The model under review builds one solid part; all positions refer to its coordinate system, in mm. A direction names the side the tool comes from. Give positions to 0.01 mm unless a question says otherwise; leave off trailing zeros. Loops run counter-clockwise (first coordinate to the right, second up) from the corner with the lowest first, then second, coordinate; pieces in that order, holes last. Notation, with made-up numbers: M -5.5,2 L 7.5,2 A4 ccw 7.5,8 Z; hole C 7.25,37.5 d2. An arc over 180 degrees is marked long. Write item = value, one per line. Start each with the question number.
1. Draft analysis for pull direction Z (two halves, no side actions). For faces 4 (the face through (48.1, 4.24, -15.86)), 5 (the face through (29, 5, -5)), 6 (the face through (6, 5, -20)), 7 (the face through (28.521, 1.774, -18.845)), state which applies: pulls with the +Z half, pulls with the -Z half, needs draft (parallel to the pull), parting line crosses it, or undercut.
2. We need section A-A on x = 53.5. Give the boundary of the cut face in (y, z), then the cut area to 4 significant figures.
3. Wall thickness on line 1 along X through (y, z) = (1.95, -20); line 2 along Y through (x, z) = (5, -16.75); line 3 along Z through (x, y) = (4, 1): over which ranges is each line inside the solid? List them lowest first. Write a range as from..to.
4. We need section D-D on x = 44. Give the boundary of the cut face in (y, z).
5. We need section B-B on z = -20. Give the boundary of the cut face in (x, y), then the cut area to 3 significant figures.
6. We need section C-C on y = 2. Give the boundary of the cut face in (x, z), then the cut area to 3 significant figures.
7. For faces 1 (the face through (45.054, 1.774, -19.328)), 2 (the face through (29, 7, -15)), 3 (the face through (52, 5, -20)), list the 3-axis set-ups (+Z, -Z, +X, -X, +Y, -Y) from which the entire face can be reached by the end or side of a thin tool; tool diameter is ignored.
8. For pin 1 (3 mm diameter, centred on x = 32.5, y = 6.5, fed in from -Z); pin 2 (11 mm diameter, centred on x = 7, z = -22, fed in from +Y); pin 3 (1.5 mm diameter, centred on x = 53.5, z = -20, fed in from +Y); pin 4 (1.5 mm diameter, centred on x = 26, y = 6, fed in from +Z), all flat-tipped, find the tip position at first contact; note any pin that passes through.
from build123d import *

# Parameters (mm, degrees)
BOSS_EXTRUDE1_DEPTH = 58
SKETCH3_W           = 40
SKETCH3_H           = 10
CUT_EXTRUDE2_DEPTH  = 6.5
CUT_EXTRUDE3_REACH  = 65.492
SKETCH4_R           = 1.25
SKETCH5_W           = 58
SKETCH5_H           = 10
CUT_EXTRUDE4_DEPTH  = 5
CUT_EXTRUDE5_REACH  = 65.356
SKETCH6_R           = 1.25
FILLET1_R           = 3


with BuildPart() as part:
    # Sketch1 → Boss-Extrude1 (new body)
    with BuildSketch(Plane(origin=(0, 0, 0), x_dir=(0, 0, -1), z_dir=(1, 0, 0))):
        Polygon((0, 0), (10, 10), (25, 10), (25, 0), align=None)
    extrude(amount=BOSS_EXTRUDE1_DEPTH)

    # Sketch3 → Cut-Extrude2 (cut)
    with BuildSketch(Plane(origin=(0, 10, 0), x_dir=(1, 0, 0), z_dir=(0, 1, 0))):
        with Locations((29, 20)):
            Rectangle(SKETCH3_W, SKETCH3_H)
    extrude(amount=-CUT_EXTRUDE2_DEPTH, mode=Mode.SUBTRACT)

    # Sketch4 → Cut-Extrude3 (cut, up to next)
    with BuildSketch(Plane(origin=(0, 3.5, 0), x_dir=(1, 0, 0), z_dir=(0, 1, 0)), mode=Mode.PRIVATE) as cut_extrude3_sk1:
        with Locations(Location((14, 20, 0), (0, 0, 270))):
            Circle(SKETCH4_R)
    cut_extrude3_tool1 = extrude(cut_extrude3_sk1.sketch, amount=-CUT_EXTRUDE3_REACH, mode=Mode.PRIVATE) & part.part
    # Sketch4 → Cut-Extrude3 (cut, up to next)
    with BuildSketch(Plane(origin=(0, 3.5, 0), x_dir=(1, 0, 0), z_dir=(0, 1, 0)), mode=Mode.PRIVATE) as cut_extrude3_sk2:
        with Locations(Location((29, 20, 0), (0, 0, 270))):
            Circle(SKETCH4_R)
    cut_extrude3_tool2 = extrude(cut_extrude3_sk2.sketch, amount=-CUT_EXTRUDE3_REACH, mode=Mode.PRIVATE) & part.part
    # Sketch4 → Cut-Extrude3 (cut, up to next)
    with BuildSketch(Plane(origin=(0, 3.5, 0), x_dir=(1, 0, 0), z_dir=(0, 1, 0)), mode=Mode.PRIVATE) as cut_extrude3_sk3:
        with Locations(Location((44, 20, 0), (0, 0, 270))):
            Circle(SKETCH4_R)
    cut_extrude3_tool3 = extrude(cut_extrude3_sk3.sketch, amount=-CUT_EXTRUDE3_REACH, mode=Mode.PRIVATE) & part.part
    add(cut_extrude3_tool1.solids().sort_by_distance((14, 3.5, -20))[0], mode=Mode.SUBTRACT)
    add(cut_extrude3_tool2.solids().sort_by_distance((29, 3.5, -20))[0], mode=Mode.SUBTRACT)
    add(cut_extrude3_tool3.solids().sort_by_distance((44, 3.5, -20))[0], mode=Mode.SUBTRACT)

    # Sketch5 → Cut-Extrude4 (cut)
    with BuildSketch(Plane(origin=(0, 10, 0), x_dir=(1, 0, 0), z_dir=(0, 1, 0))):
        with Locations((29, 20)):
            Rectangle(SKETCH5_W, SKETCH5_H)
    extrude(amount=-CUT_EXTRUDE4_DEPTH, mode=Mode.SUBTRACT)

    # Sketch6 → Cut-Extrude5 (cut, up to next)
    with BuildSketch(Plane(origin=(0, 5, 0), x_dir=(1, 0, 0), z_dir=(0, 1, 0)), mode=Mode.PRIVATE) as cut_extrude5_sk1:
        with Locations(Location((4.5, 20, 0), (0, 0, 270))):
            Circle(SKETCH6_R)
    cut_extrude5_tool1 = extrude(cut_extrude5_sk1.sketch, amount=-CUT_EXTRUDE5_REACH, mode=Mode.PRIVATE) & part.part
    # Sketch6 → Cut-Extrude5 (cut, up to next)
    with BuildSketch(Plane(origin=(0, 5, 0), x_dir=(1, 0, 0), z_dir=(0, 1, 0)), mode=Mode.PRIVATE) as cut_extrude5_sk2:
        with Locations(Location((53.5, 20, 0), (0, 0, 270))):
            Circle(SKETCH6_R)
    cut_extrude5_tool2 = extrude(cut_extrude5_sk2.sketch, amount=-CUT_EXTRUDE5_REACH, mode=Mode.PRIVATE) & part.part
    add(cut_extrude5_tool1.solids().sort_by_distance((4.5, 5, -20))[0], mode=Mode.SUBTRACT)
    add(cut_extrude5_tool2.solids().sort_by_distance((53.5, 5, -20))[0], mode=Mode.SUBTRACT)

    # Fillet1
    fillet1_edges = [part.edges().sort_by_distance(p)[0] for p in [
        (9, 4.25, -15),
        (49, 4.25, -15),
    ]]
    fillet(fillet1_edges, radius=FILLET1_R)


solid = part.part
Final values:
q1.face_4 = pulls with the -Z half
q1.face_5 = pulls with the +Z half
q1.face_6 = needs draft
q1.face_7 = undercut
q2.outline = M 0,-25 L 5,-25 L 5,-21.25 L 0,-21.25 Z; M 0,-18.75 L 5,-18.75 L 5,-15 L 10,-15 L 10,-10 L 0,0 Z
q2.area = 137.5 mm²
q3.line_1 = 0..3.25, 5.75..12.75, 15.25..27.75, 30.25..42.75, 45.25..52.25, 54.75..58
q3.line_2 = 0..5
q3.line_3 = -25..-21.15, -18.85..-1
q4.outline = M 0,-25 L 3.5,-25 L 3.5,-21.25 L 0,-21.25 Z; M 0,-18.75 L 3.5,-18.75 L 3.5,-15 L 10,-15 L 10,-10 L 0,0 Z
q5.outline = M 0,0 L 3.25,0 L 3.25,5 L 0,5 Z; M 5.75,0 L 12.75,0 L 12.75,3.5 L 9,3.5 L 9,5 L 5.75,5 Z; M 15.25,0 L 27.75,0 L 27.75,3.5 L 15.25,3.5 Z; M 30.25,0 L 42.75,0 L 42.75,3.5 L 30.25,3.5 Z; M 45.25,0 L 52.25,0 L 52.25,5 L 49,5 L 49,3.5 L 45.25,3.5 Z; M 54.75,0 L 58,0 L 58,5 L 54.75,5 Z
q5.area = 179 mm²
q6.outline = M 0,-25 L 58,-25 L 58,-2 L 0,-2 Z; hole C 4.5,-20 d2.5; hole C 14,-20 d2.5; hole C 29,-20 d2.5; hole C 44,-20 d2.5; hole C 53.5,-20 d2.5
q6.area = 1,310 mm²
q7.face_1 = +Y, -Y
q7.face_2 = -Z, +Y
q7.face_3 = -Z, +X, -X, +Y
q8.pin_1 = -15
q8.pin_2 = 5
q8.pin_3 = through
q8.pin_4 = -5.25
